```python
from build123d import *

# Parameters (mm, degrees)
F1_DEPTH = 8
F2_R     = 6
F3_DEPTH = 25
F4_R     = 4
F5_DEPTH = 4
F6_R     = 4
F7_DEPTH = 6


with BuildPart() as f1:
    # F0 (on Top) → F1 (new body)
    with BuildSketch(Plane.XY):
        Polygon((8.878189, 1.303729), (7.873311, 1.156166), (7.39657, 2.935387), (8.340604, 3.310035), (8.822399, 3.654358), (9.885736, 5.137187), (9.391802, 5.992704), (7.575968, 5.813244), (7.036875, 5.568157), (6.240405, 4.937924), (4.937924, 6.240405), (5.568157, 7.036876), (5.813244, 7.575967), (5.992704, 9.391803), (5.137187, 9.885737), (3.654357, 8.822399), (3.310035, 8.340604), (2.935388, 7.39657), (1.156166, 7.873311), (1.303728, 8.878189), (1.246434, 9.467602), (0.493934, 11.129891), (-0.493934, 11.129891), (-1.246434, 9.467602), (-1.303728, 8.878189), (-1.156166, 7.873311), (-2.935388, 7.39657), (-3.310035, 8.340604), (-3.654357, 8.822399), (-5.137187, 9.885737), (-5.992704, 9.391803), (-5.813244, 7.575967), (-5.568157, 7.036876), (-4.937924, 6.240405), (-6.240405, 4.937924), (-7.036875, 5.568157), (-7.575968, 5.813244), (-9.391802, 5.992704), (-9.885736, 5.137187), (-8.822399, 3.654358), (-8.340604, 3.310035), (-7.39657, 2.935387), (-7.873311, 1.156166), (-8.878189, 1.303729), (-9.467602, 1.246434), (-11.129891, 0.493934), (-11.129891, -0.493934), (-9.467602, -1.246434), (-8.878189, -1.303729), (-7.873311, -1.156165), (-7.39657, -2.935387), (-8.340604, -3.310035), (-8.822399, -3.654358), (-9.885736, -5.137186), (-9.391802, -5.992704), (-7.575968, -5.813244), (-7.036875, -5.568156), (-6.240405, -4.937924), (-4.937924, -6.240405), (-5.568157, -7.036876), (-5.813244, -7.575967), (-5.992704, -9.391803), (-5.137187, -9.885737), (-3.654357, -8.822399), (-3.310035, -8.340603), (-2.935388, -7.39657), (-1.156166, -7.873311), (-1.303728, -8.878188), (-1.246434, -9.467602), (-0.493934, -11.12989), (0.493934, -11.12989), (1.246434, -9.467602), (1.303728, -8.878188), (1.156166, -7.873311), (2.935388, -7.39657), (3.310035, -8.340603), (3.654357, -8.822399), (5.137187, -9.885737), (5.992704, -9.391803), (5.813244, -7.575967), (5.568157, -7.036876), (4.937924, -6.240405), (6.240405, -4.937924), (7.036875, -5.568156), (7.575968, -5.813244), (9.391802, -5.992704), (9.885736, -5.137186), (8.822399, -3.654358), (8.340604, -3.310035), (7.39657, -2.935387), (7.873311, -1.156165), (8.878189, -1.303729), (9.467602, -1.246434), (11.12989, -0.493934), (11.12989, 0.493934), (9.467602, 1.246434), align=None)
    extrude(amount=F1_DEPTH)

    # F2 (on face) → F3 (join)
    with BuildSketch(Plane.XY.offset(8)):
        Circle(F2_R)
    extrude(amount=F3_DEPTH)

    # F4 (on face) → F5 (join)
    with BuildSketch(Plane(origin=(0, 0, 0), x_dir=(1, 0, 0), z_dir=(0, 0, -1))):
        Circle(F4_R)
    extrude(amount=F5_DEPTH)

    # F6 (on Front) → F7 (cut, symmetric)
    with BuildSketch(Plane.XZ):
        with Locations((0, 25)):
            Circle(F6_R)
    extrude(amount=F7_DEPTH, both=True, mode=Mode.SUBTRACT)


solid = f1.part
```
Source: CAD feature listing. Evaluate the final solid. Frame: model axes, mm. A direction names the side the tool comes from. Coordinates: 2 decimals unless noted, no trailing zeros. Write each loop counter-clockwise with the first axis right and the second up, starting at its lowest first coordinate (ties: lowest second). Pieces come first, ordered by that corner, then holes. Notation, with made-up numbers: (-27, 14) -> (22, 14) arc R7 ccw to (22, 26) -> close; hole circle Ø11 at (-24, 54.5). An arc over 180 degrees is marked (long way). Return JSON: item names as keys, results as strings. Group by question number.
1) Section query D-D, the plane z = 23.5. Return loops of the section in (x, y).
2) Section query A-A, the plane x = 0. Return loops of the section in (y, z).
3) Contact query for flat-ended pins moving along their axis: P1, Ø1.5, axis at y = 3, z = 12.5, coming from the -X side; P2, Ø8, axis at x = -3.5, z = 23.5, coming from the +Y side; P3, Ø2, axis at x = -1, y = 5.5, coming from the -Z side; P4, Ø6.5, axis at x = 0, z = 25, coming from the -Y side. Output: stop coordinate, or through.
4) Section query C-C, the plane z = 13. Return loops of the section in (x, y).
5) Ray query, line 1 along X through (y, z) = (-0.25, 25); line 2 along X through (y, z) = (1.5, 25); line 3 along Z through (x, y) = (0, -2.75). Return the intervals inside material, ascending.
6) Section query B-B, the plane y = 0. Return loops of the section in (x, z), plus the area to 3 significant figures.
7) Mould query, pull axis X, two halves, no side actions, for faces 1 (the face through (8.497, 5.904, 3.944)), 2 (the face through (-6, 0, 20)), 3 (the face through (9.64, 5.56, 3.94)). Classes: +X half, -X half, draft (parallel to the pull), parting line (faces both ways), or undercut.
8) Set-up query: faces 4 (the face through (-7.875, 3.125, 3.944)), 5 (the face through (-8.497, -5.904, 3.944)), 6 (the face through (-5.58, 5.6, 3.94)). Return all of +Z, -Z, +X, -X, +Y, -Y with unobstructed straight access to the full face (end or side cutting, diameter ignored); none if empty.
From the geometry:
{
 "1": {"outline": "(-3.71, -4.72) -> (-3.71, 4.72) arc R6 ccw to start; (3.71, -4.72) arc R6 ccw to (3.71, 4.72) -> close"},
 "2": {"outline": "(-11.13, 0) -> (-4, 0) -> (-4, -4) -> (4, -4) -> (4, 0) -> (11.13, 0) -> (11.13, 8) -> (6, 8) -> (6, 21) -> (-6, 21) -> (-6, 8) -> (-11.13, 8) -> close; (-6, 29) -> (6, 29) -> (6, 33) -> (-6, 33) -> close"},
 "3": {"P1": "x = -5.56", "P2": "y = 5.99", "P3": "z = 0", "P4": "through"},
 "4": {"outline": "circle Ø12 at (0, 0)"},
 "5": {"line 1": "-5.99 to -4, 4 to 5.99", "line 2": "-5.81 to -4, 4 to 5.81", "line 3": "-4 to 21, 29 to 33"},
 "6": {"outline": "(-11.13, 0) -> (-4, 0) -> (-4, -4) -> (4, -4) -> (4, 0) -> (11.13, 0) -> (11.13, 8) -> (6, 8) -> (6, 33) -> (-6, 33) -> (-6, 8) -> (-11.13, 8) -> close; hole circle Ø8 at (0, 25)", "area": "460 mm²"},
 "7": {"face 1": "undercut", "face 2": "parting line", "face 3": "+X half"},
 "8": {"face 4": "+Z, -Z, -X", "face 5": "+Z, -Z, -Y", "face 6": "+Z, -Z"}
}
